Geometry: final body of the model. Coordinates: model frame, mm. Face numbers are marked on the shaded views. Round coordinates to 2 decimals unless told otherwise and drop trailing zeros. Loops run counter-clockwise (first coordinate to the right, second up) from the corner with the lowest first, then second, coordinate; pieces in that order, holes last. Notation, with made-up numbers: (25.5, 51) -> (37.5, 51) arc R25 ccw to (37.5, 82) -> close; hole circle Ø2 at (3.25, 11). An arc over 180 degrees is marked (long way). Answer in a Markdown table with one row per item.
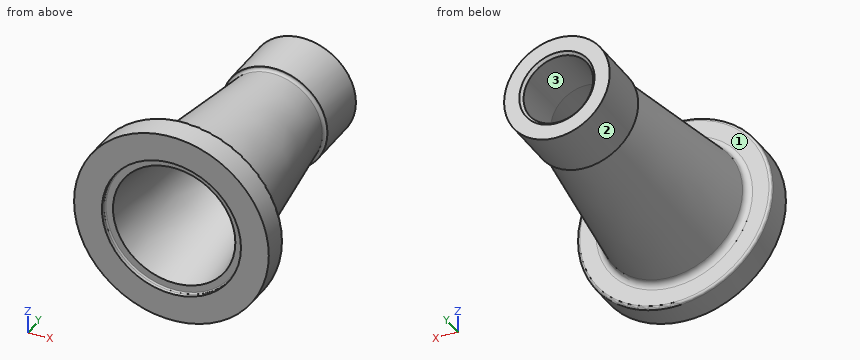
```python
from build123d import *

# Parameters (mm, degrees)
FILLET1_R     = 5
CHAMFER1_SIZE = 2
FILLET2_R     = 1
FILLET3_R     = 2
FILLET4_R     = 2


with BuildPart() as part:
    # Sketch1 → Revolve1 (revolve)
    with BuildSketch(Plane.XY):
        Polygon((50, -88.657309004), (50, -92.5), (70, -92.5), (70, -72.5), (51.919566163, -72.5), (35.129649231, 52.5), (38, 52.5), (38, 92.5), (25.03984406, 92.5), (25.03984406, 90.5), (25.03984406, 52.5), (44, -88.657309004), align=None)
    revolve(axis=Axis((0, -92.5, 0), (0, 1, 0)))

    # Fillet1
    fillet1_edges = [part.edges().sort_by_distance(p)[0] for p in [
        (-51.919566163, -72.5, 0),
    ]]
    fillet(fillet1_edges, radius=FILLET1_R)

    # Chamfer1
    chamfer1_edges = [part.edges().sort_by_distance(p)[0] for p in [
        (-25.03984406, 92.5, 0),
    ]]
    chamfer(chamfer1_edges, length=CHAMFER1_SIZE)

    # Fillet2
    fillet2_edges = [part.edges().sort_by_distance(p)[0] for p in [
        (-50, -88.657309004, 0),
    ]]
    fillet(fillet2_edges, radius=FILLET2_R)

    # Fillet3
    fillet3_edges = [part.edges().sort_by_distance(p)[0] for p in [
        (-70, -72.5, 0),
    ]]
    fillet(fillet3_edges, radius=FILLET3_R)

    # Fillet4
    fillet4_edges = [part.edges().sort_by_distance(p)[0] for p in [
        (-35.129649231, 52.5, 0),
    ]]
    fillet(fillet4_edges, radius=FILLET4_R)


solid = part.part
```
Item 1: Mould query, pull axis Z, two halves, no side actions, for the marked faces 1, 2 and 3. Classes: released by +Z, released by -Z, zero draft, split by the parting line, or undercut.
Ans:
| item | result |
|---|---|
| face 1 | zero draft |
| face 2 | split by the parting line |
| face 3 | undercut |
Item 2: First-contact query: P1, Ø6, axis at x = -27, y = -39, coming from the -Z side; P2, Ø5, axis at y = 44.5, z = -24.5, coming from the +X side; P3, Ø10, axis at x = 38, z = -21, coming from the -Y side. Flat tips, straight axial feed; report the tip coordinate or a pass-through.
Ans:
| item | result |
|---|---|
| P1 | z = -40.96 |
| P2 | x = 28.8 |
| P3 | y = -88.66 |
Item 3: Ray query, L1, parallel to X at y = 77, z = 0; L2, parallel to X at y = -90, z = 0. Return the intervals inside material, ascending.
Ans:
| item | result |
|---|---|
| L1 | -38 to -25.04, 25.04 to 38 |
| L2 | -70 to -50, 50 to 70 |
Item 4: Section query C-C, the plane y = 70. Output: boundary loops of the cut face in (x, z), and give its area (3 significant figures).
Ans:
| item | result |
|---|---|
| outline | circle Ø76 at (0, 0); hole circle Ø50.08 at (0, 0) |
| area | 2,570 mm2 |
